```python
from build123d import *

# Parameters (mm, degrees)
SM_BASE_FLANGE_1_DEPTH = 1.5
OTHER_START            = -16
OTHER_1_DEPTH          = 32
OTHER_1_2_DEPTH        = 32
OTHER_START_2          = -18
OTHER_1_3_DEPTH        = 36
SKETCH_7_R             = 1
CUT_EXTRUDE_1_DEPTH    = 40.796735326
SKETCH_8_R             = 4
SKETCH_8_R_2           = 0.95
CUT_EXTRUDE_2_DEPTH    = 10


with BuildPart() as part:
    # 基体-法兰1: sheet metal written as solids
    # Sketch 1 → 基体-法兰1 (new body)
    with BuildSketch(Plane.XY):
        with BuildLine():
            Line((-24, -16), (24, -16))
            ThreePointArc((24, -16), (26.121320344, -15.121320344), (27, -13))
            Line((27, -13), (27, 13))
            ThreePointArc((27, 13), (26.121320344, 15.121320344), (24, 16))
            Line((24, 16), (-24, 16))
            ThreePointArc((-24, 16), (-26.121320344, 15.121320344), (-27, 13))
            Line((-27, 13), (-27, -13))
            ThreePointArc((-27, -13), (-26.121320344, -15.121320344), (-24, -16))
        make_face()
    extrude(amount=-SM_BASE_FLANGE_1_DEPTH)

    # Other 1: read off the stored shape, not the designer's step
    # Other 1 outline → Other 1 (cut)
    with BuildSketch(Plane(origin=(0, 0, 0), x_dir=(1, 0, 0), z_dir=(0, 1, 0)).offset(OTHER_START)):
        with BuildLine():
            ThreePointArc((-17.375223856, 0), (-16.558564082, 1.086838938), (-15.2634, 1.5))
            Line((-15.2634, 1.5), (-27, 1.5))
            Line((-27, 1.5), (-27, 0))
            Line((-27, 0), (-17.375223856, 0))
        make_face()
        with BuildLine():
            Line((27, 1.5), (15.2634, 1.5))
            ThreePointArc((15.2634, 1.5), (16.558564082, 1.086838938), (17.375223856, 0))
            Line((17.375223856, 0), (27, 0))
            Line((27, 0), (27, 1.5))
        make_face()
    extrude(amount=OTHER_1_DEPTH, mode=Mode.SUBTRACT)

    # Other 1 2 outline → Other 1 2 (add)
    with BuildSketch(Plane(origin=(0, 0, 0), x_dir=(1, 0, 0), z_dir=(0, 1, 0)).offset(OTHER_START)):
        with BuildLine():
            Line((-15.2634, 0), (-17.375223856, 0))
            ThreePointArc((-17.375223856, 0), (-17.468585343, -0.363053267), (-17.5, -0.7366))
            Line((-17.5, -0.7366), (-17.5, -10.138054181))
            Line((-17.5, -10.138054181), (-16, -10.138054181))
            Line((-16, -10.138054181), (-16, -0.7366))
            ThreePointArc((-16, -0.7366), (-15.784254855, -0.215745145), (-15.2634, 0))
        make_face()
        with BuildLine():
            ThreePointArc((17.5, -0.7366), (17.468585343, -0.363053267), (17.375223856, 0))
            Line((17.375223856, 0), (15.2634, 0))
            ThreePointArc((15.2634, 0), (15.784254855, -0.215745145), (16, -0.7366))
            Line((16, -0.7366), (16, -10.138054181))
            Line((16, -10.138054181), (17.5, -10.138054181))
            Line((17.5, -10.138054181), (17.5, -0.7366))
        make_face()
    extrude(amount=OTHER_1_2_DEPTH)

    # Other 1 3 outline → Other 1 3 (cut)
    with BuildSketch(Plane.YZ.offset(OTHER_START_2)):
        with BuildLine():
            ThreePointArc((-16, 7.138054181), (-15.121320344, 9.259374525), (-13, 10.138054181))
            Line((-13, 10.138054181), (-16, 10.138054181))
            Line((-16, 10.138054181), (-16, 7.138054181))
        make_face()
        with BuildLine():
            ThreePointArc((13, 10.138054181), (15.121320344, 9.259374525), (16, 7.138054181))
            Line((16, 7.138054181), (16, 10.138054181))
            Line((16, 10.138054181), (13, 10.138054181))
        make_face()
    extrude(amount=OTHER_1_3_DEPTH, mode=Mode.SUBTRACT)

    # 草图7 → 切除-拉伸1 (cut, through all)
    with BuildSketch(Plane.ZY.offset(17.5)):
        with Locations((7.638054181, 8)):
            Circle(SKETCH_7_R)
        with Locations((7.638054181, -8)):
            Circle(SKETCH_7_R)
    extrude(amount=-CUT_EXTRUDE_1_DEPTH, mode=Mode.SUBTRACT)

    # 草图8 → 切除-拉伸2 (cut)
    with BuildSketch(Plane.XY):
        Circle(SKETCH_8_R)
        with Locations((0, 8)):
            Circle(SKETCH_8_R_2)
        with Locations((8, 0)):
            Circle(SKETCH_8_R_2)
        with Locations((0, -8)):
            Circle(SKETCH_8_R_2)
        with Locations((-8, 0)):
            Circle(SKETCH_8_R_2)
    extrude(amount=-CUT_EXTRUDE_2_DEPTH, mode=Mode.SUBTRACT)


solid = part.part
```
Can you work these out from the model? Positions are in its coordinate system, mm. A direction names the side the tool comes from. Round coordinates to 2 decimals unless told otherwise and drop trailing zeros. Loops run counter-clockwise (first coordinate to the right, second up) from the corner with the lowest first, then second, coordinate; pieces in that order, holes last. Notation, with made-up numbers: M -36,-37 L -4,-37 A7 ccw -4,-32 Z; hole C 68.25,37 d10. An arc over 180 degrees is marked long. Write item = value, one per line. Start each with the question number.
(1) If we mould it in two halves opening along Z, with no side actions, what happens to faces 1 (the face through (16.74, 8.99, 7.51)), 2 (the face through (17.5, 0, 6)), 3 (the face through (16.74, -15.14, 9.24))? For each: released by +Z, released by -Z, zero draft, split by the parting line, or undercut.
(2) Suppose I cut it at C-C on x = 8. Write out the boundary of the cut face in (y, z), plus the area to 4 significant figures.
(3) I'm going to push flat-ended pins straight in: P1, Ø1.5, axis at x = 0, y = -8, coming from the -Z side; P2, Ø3, axis at x = 0, y = 8, coming from the -Z side; P3, Ø3, axis at x = 13.5, y = -2.5, coming from the +Z side. Where does each tip first touch, or does it pass through?
(4) Suppose I cut it at D-D on y = 9.5. Write out the boundary of the cut face in (x, z).
(5) Suppose I cut it at A-A on z = 4.25. Write out the boundary of the cut face in (x, y), plus the area to 3 significant figures.
(6) I need wall thicknesses on line 1 along X through (y, z) = (-7.5, 3); line 2 along Z through (x, y) = (-2, 12); line 3 along Y through (x, z) = (8, -0.8). Which ranges of each line are inside material? Lowest first, please.
(7) Suppose I cut it at B-B on y = 0. Write out the boundary of the cut face in (x, z).
(8) Which directions (+Z, -Z, +X, -X, +Y, -Y) give clear straight access to the entire face, cutting with the end or side of a thin tool? Please do faces 4 (the face through (-16, 0, 6)), 5 (the face through (-17.5, 0, 5)).
Answer block:
q1.face_1 = undercut
q1.face_2 = zero draft
q1.face_3 = released by +Z
q2.outline = M -16,-1.5 L -0.95,-1.5 L -0.95,0 L -16,0 Z; M 0.95,-1.5 L 16,-1.5 L 16,0 L 0.95,0 Z
q2.area = 45.15 mm²
q3.P1 = through
q3.P2 = -1.5
q3.P3 = 0
q4.outline = M -17.5,0.74 A2.24 ccw -15.26,-1.5 L 15.26,-1.5 A2.24 ccw 17.5,0.74 L 17.5,10.14 L 16,10.14 L 16,0.74 A0.74 cw 15.26,0 L -15.26,0 A0.74 cw -16,0.74 L -16,10.14 L -17.5,10.14 Z
q5.outline = M -17.5,-16 L -16,-16 L -16,16 L -17.5,16 Z; M 16,-16 L 17.5,-16 L 17.5,16 L 16,16 Z
q5.area = 96.0 mm²
q6.line_1 = -17.5 to -16, 16 to 17.5
q6.line_2 = -1.5 to 0
q6.line_3 = -16 to -0.95, 0.95 to 16
q7.outline = M -17.5,0.74 A2.24 ccw -15.26,-1.5 L -8.95,-1.5 L -8.95,0 L -15.26,0 A0.74 cw -16,0.74 L -16,10.14 L -17.5,10.14 Z; M -7.05,-1.5 L -4,-1.5 L -4,0 L -7.05,0 Z; M 4,-1.5 L 7.05,-1.5 L 7.05,0 L 4,0 Z; M 8.95,-1.5 L 15.26,-1.5 A2.24 ccw 17.5,0.74 L 17.5,10.14 L 16,10.14 L 16,0.74 A0.74 cw 15.26,0 L 8.95,0 Z
q8.face_4 = +Z, +Y, -Y
q8.face_5 = +Z, -Z, -X, +Y, -Y
